```python
from build123d import *

# Parameters (mm, degrees)
SKETCH2_W           = 200
SKETCH2_H           = 85
BOSS_EXTRUDE1_DEPTH = 70
SKETCH3_W           = 51
SKETCH3_H           = 51
CUT_EXTRUDE1_DEPTH  = 229.309001137
FILLET1_R           = 5
SKETCH4_R           = 6.415
CUT_EXTRUDE2_DEPTH  = 229.309001137


with BuildPart() as part:
    # Sketch2 → Boss-Extrude1 (new body)
    with BuildSketch(Plane.XY):
        with Locations((100, 42.5)):
            Rectangle(SKETCH2_W, SKETCH2_H)
    extrude(amount=BOSS_EXTRUDE1_DEPTH)

    # Sketch3 → Cut-Extrude1 (cut, through all)
    with BuildSketch(Plane(origin=(200, 0, 0), x_dir=(0, 0, -1), z_dir=(1, 0, 0))):
        with Locations((-35, 25.5)):
            Rectangle(SKETCH3_W, SKETCH3_H)
    extrude(amount=-CUT_EXTRUDE1_DEPTH, mode=Mode.SUBTRACT)

    # Fillet1
    fillet1_edges = [part.edges().sort_by_distance(p)[0] for p in [
        (100, 0, 0),
        (100, 0, 70),
    ]]
    fillet(fillet1_edges, radius=FILLET1_R)

    # Sketch4 → Cut-Extrude2 (cut, through all)
    with BuildSketch(Plane.XY.offset(70)):
        with Locations((125, 73.585)):
            Circle(SKETCH4_R)
        with Locations(Location((75, 73.585, 0), (0, 0, 180))):
            Circle(SKETCH4_R)
    extrude(amount=-CUT_EXTRUDE2_DEPTH, mode=Mode.SUBTRACT)


solid = part.part
```
Design review of the part built by this model. Coordinates are the model's own, in mm. A direction names the side the tool comes from. Coordinates: 2 decimals unless noted, no trailing zeros. Order: outer loops, then holes, each group sorted by start corner. A loop starts at its lowest first (then second) coordinate and runs counter-clockwise, first axis right, second up.
1) Wall thickness on line 1 along Y through (x, z) = (75, 46); line 2 along Z through (x, y) = (102, 12); line 3 along X through (y, z) = (77, 54): over which ranges is each line inside the solid? List them lowest first.
2) Take a section at C-C, the plane z = 45. Give the boundary of the cut face in (x, y) (3 decimals), and give its area (3 significant figures).
3) Take a section at B-B, the plane x = 31.5. Give the boundary of the cut face in (y, z).
4) Take a section at A-A, the plane x = 125. Give the boundary of the cut face in (y, z).
5) Mouldability with a two-part tool opening along Z and no side actions: class faces 3 (the cylindrical face through (79.73, 69.25, 35.49)), 4 (the flat face through (101, 51, 35)), 5 (the cylindrical face through (101, 2, 1)) as +Z half, -Z half, draft (parallel to the pull), parting line (faces both ways), or undercut.
6) Clearance check with flat-ended pins moving along their axes: pin 1 (15.5 mm diameter, centred on x = 123.5, z = 29.5, fed in from -Y); pin 2 (10.5 mm diameter, centred on x = 125, y = 73.585, fed in from +Z). State where each tip first meets the part, or that it passes through.
7) For faces 1 (the flat face through (101, 25, 9.5)), 2 (the flat face through (200, 61, 35)), list the 3-axis set-ups (+Z, -Z, +X, -X, +Y, -Y) from which the entire face can be reached by the end or side of a thin tool; tool diameter is ignored.
Returned:
1. line 1: y = 51 to 67.17, 80 to 85
1. line 2: z = 0 to 9.5, 60.5 to 70
1. line 3: x = 0 to 69.57, 80.43 to 119.57, 130.43 to 200
2. outline: (0, 51) - (200, 51) - (200, 85) - (0, 85) - close; hole circle Ø12.83 at (75, 73.585); hole circle Ø12.83 at (125, 73.585)
2. area: 6,540 mm2
3. outline: (0, 5) arc R5 ccw to (5, 0) - (85, 0) - (85, 70) - (5, 70) arc R5 ccw to (0, 65) - (0, 60.5) - (51, 60.5) - (51, 9.5) - (0, 9.5) - close
4. outline: (0, 5) arc R5 ccw to (5, 0) - (67.17, 0) - (67.17, 70) - (5, 70) arc R5 ccw to (0, 65) - (0, 60.5) - (51, 60.5) - (51, 9.5) - (0, 9.5) - close; (80, 0) - (85, 0) - (85, 70) - (80, 70) - close
5. face 3: draft
5. face 4: undercut
5. face 5: -Z half
6. pin 1: stops at y = 51
6. pin 2: passes through
7. face 1: +X, -X, -Y
7. face 2: +Z, -Z, +X, +Y, -Y
